```python
from build123d import *

# Parameters (mm, degrees)
BOSS_EXTRUDE1_DEPTH = 1.5875
SKETCH7_R           = 52.705
SKETCH7_R_2         = 44.45
CUT_EXTRUDE1_DEPTH  = 20.32


with BuildPart() as part:
    # Sketch3 → Boss-Extrude1 (new body, symmetric)
    with BuildSketch(Plane(origin=(0, 0, 0), x_dir=(1, 0, 0), z_dir=(0, 1, 0))):
        Polygon((-279.4, 95.25), (-139.7, 95.25), (-120.65, 133.35), (133.35, 133.35), (152.4, 95.25), (279.4, 95.25), (279.4, -95.25), (152.4, -95.25), (133.35, -133.35), (-120.65, -133.35), (-139.7, -95.25), (-279.4, -95.25), align=None)
    extrude(amount=BOSS_EXTRUDE1_DEPTH, both=True)

    # Sketch7 → Cut-Extrude1 (cut)
    with BuildSketch(Plane(origin=(0, 1.5875, 0), x_dir=(1, 0, 0), z_dir=(0, 1, 0))):
        with Locations((89.349601684, 0)):
            Circle(SKETCH7_R)
        with Locations((201.029841253, -5.49358251)):
            Circle(SKETCH7_R_2)
    extrude(amount=-CUT_EXTRUDE1_DEPTH, mode=Mode.SUBTRACT)


solid = part.part
```
Work out the finished part from the listing and answer in its coordinate system (mm). Coordinates: 2 decimals unless noted, no trailing zeros. Loops run counter-clockwise (first coordinate to the right, second up) from the corner with the lowest first, then second, coordinate; pieces in that order, holes last.
1) Flat-ended cylindrical pins translate along their axes: pin 1 (1.5 mm diameter, centred on x = -223.5, y = 0, fed in from +Z); pin 2 (1.6 mm diameter, centred on x = 200, y = 0.5, fed in from -Z). Find the tip coordinate at first contact, or state that the pin passes through.
Results:
pin 1: stops at z = 95.25
pin 2: stops at z = -95.25
2) Section A-A (z = -10) is taken. Give the vertices of the cut face in (x, y), plus the area to 3 significant figures.
Results:
outline: (-279.4, -1.59) - (37.6, -1.59) - (37.6, 1.59) - (-279.4, 1.59) - close; (141.1, -1.59) - (159.37, -1.59) - (159.37, 1.59) - (141.1, 1.59) - close; (242.69, -1.59) - (279.4, -1.59) - (279.4, 1.59) - (242.69, 1.59) - close
area: 1,180 mm2
3) Section B-B (x = 108.5) is taken. Give the vertices of the cut face in (y, z).
Results:
outline: (-1.59, -133.35) - (1.59, -133.35) - (1.59, -49.1) - (-1.59, -49.1) - close; (-1.59, 49.1) - (1.59, 49.1) - (1.59, 133.35) - (-1.59, 133.35) - close
4) For a pull along X with two mould halves and no side action, classify faces 1 (the flat face through (4, -1.588, -2)), 2 (the cylindrical face through (138.036, 0.022, 20.186)), 3 (the flat face through (-130.04, 0.02, 114.57)) as +X half, -X half, draft (parallel to the pull), parting line (faces both ways), or undercut.
Results:
face 1: draft
face 2: undercut
face 3: -X half
5) Section C-C (z = -45.5) is taken. Give the vertices of the cut face in (x, y), plus the area to 3 significant figures.
Results:
outline: (-279.4, -1.59) - (62.75, -1.59) - (62.75, 1.59) - (-279.4, 1.59) - close; (115.95, -1.59) - (279.4, -1.59) - (279.4, 1.59) - (115.95, 1.59) - close
area: 1,610 mm2
6) Section D-D (x = -195.5) is taken. Give the vertices of the cut face in (y, z).
Results:
outline: (-1.59, -95.25) - (1.59, -95.25) - (1.59, 95.25) - (-1.59, 95.25) - close
7) Consider probe 1 along Z at (x, y) = (87.5, -0.05); probe 2 along X at (y, z) = (1.1, 37.5); probe 3 along X at (y, z) = (-0.15, 0). Determine where each line is inside the solid, lowest interval first.
Results:
probe 1: z = -133.35 to -52.67, 52.67 to 133.35
probe 2: x = -279.4 to 52.31, 126.38 to 170.19, 231.87 to 279.4
probe 3: x = -279.4 to 36.64, 142.05 to 156.92, 245.14 to 279.4
